Model file for the job. Use its own axes, mm. Face numbers are marked on the shaded views. A direction names the side the tool comes from. Round coordinates to 2 decimals unless told otherwise and drop trailing zeros. Order: outer loops, then holes, each group sorted by start corner. A loop starts at its lowest first (then second) coordinate and runs counter-clockwise, first axis right, second up. Notation, with made-up numbers: M 76,-0.75 L 126,-0.75 A29 cw 126,33.25 Z; hole C 23.25,72.5 d8. An arc over 180 degrees is marked long. Return JSON: item names as keys, results as strings. Group by question number.
Item 1: Slice it at A-A on y = 171.5. Write the cut outline in (x, z), then the cut area to 3 significant figures.
Item 2: Pin check, flat tips, straight feed: pin 1 Ø2 at (x, y) = (-13.5, 445.5) entering from +Z; pin 2 Ø1 at (x, y) = (-13, 370.5) entering from -Z; pin 3 Ø8 at (x, y) = (25.5, 67) entering from +Z. Stop position of each tip, or through.
Item 3: Which spindle directions (+Z, -Z, +X, -X, +Y, -Y) get a long thin tool onto all of the face, cutting with end or side? Do the marked faces 1 and 2. Say none if no direction does.
Item 4: Probe line 1 along X through (y, z) = (199, -51); line 2 along Y through (x, z) = (69.5, 10); line 3 along X through (y, z) = (50.5, -37.5). List the from-to ranges inside material, lowest first.
from build123d import *

# Parameters (mm, degrees)
SKETCH1_R           = 150
BOSS_EXTRUDE1_DEPTH = 500
SKETCH2_R           = 150
SKETCH2_R_2         = 90
CUT_EXTRUDE1_DEPTH  = 400
FILLET1_R           = 100


with BuildPart() as part:
    # Sketch1 → Boss-Extrude1 (new body)
    with BuildSketch(Plane(origin=(0, 0, 0), x_dir=(1, 0, 0), z_dir=(0, 1, 0))):
        with Locations(Location((0, 0, 0), (0, 0, 270))):
            Circle(SKETCH1_R)
    extrude(amount=BOSS_EXTRUDE1_DEPTH)

    # Sketch2 → Cut-Extrude1 (cut)
    with BuildSketch(Plane.XZ):
        with Locations(Location((0, 0, 0), (0, 0, 270))):
            Circle(SKETCH2_R)
        with Locations(Location((0, 0, 0), (0, 0, 270))):
            Circle(SKETCH2_R_2, mode=Mode.SUBTRACT)
    extrude(amount=-CUT_EXTRUDE1_DEPTH, mode=Mode.SUBTRACT)

    # Fillet1
    fillet1_edges = [part.edges().sort_by_distance(p)[0] for p in [
        (0, 500, -150),
    ]]
    fillet(fillet1_edges, radius=FILLET1_R - 0.0001)  # a hair under: the kernel refuses the full size


solid = part.part
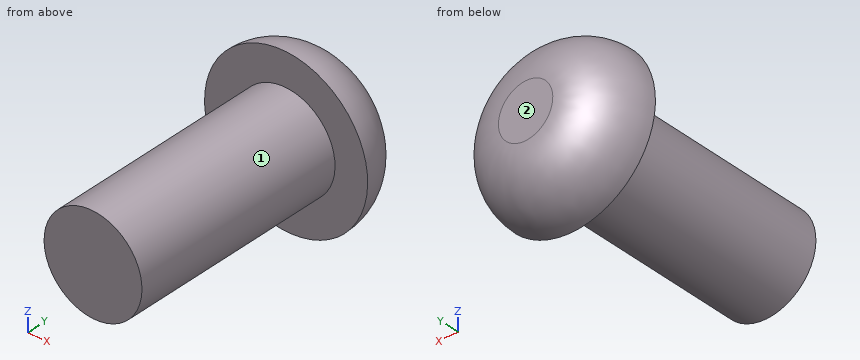
Output values:
{
 "1": {"outline": "C 0,0 d180", "area": "25,400 mm²"},
 "2": {"pin 1": "z = 138.91", "pin 2": "z = -89.13", "pin 3": "z = 87.39"},
 "3": {"face 1": "-Y", "face 2": "+Z, -Z, +X, -X, +Y"},
 "4": {"line 1": "-74.16 to 74.16", "line 2": "0 to 497.94", "line 3": "-81.82 to 81.82"}
}
